```python
from build123d import *

# Parameters (mm, degrees)
F0_W     = 60
F0_H     = 40
F0_R     = 1.75
F0_W_2   = 29
F0_H_2   = 22
F1_DEPTH = 3
F2_R     = 5


with BuildPart() as f1:
    # F0 (on Top) → F1 (new body)
    with BuildSketch(Plane.XY):
        Rectangle(F0_W, F0_H)
        with Locations((-25, 0)):
            Circle(F0_R, mode=Mode.SUBTRACT)
        Rectangle(F0_W_2, F0_H_2, mode=Mode.SUBTRACT)
        with Locations((25, 0)):
            Circle(F0_R, mode=Mode.SUBTRACT)
    extrude(amount=F1_DEPTH)

    # F2
    f2_edges = [f1.edges().sort_by_distance(p)[0] for p in [
        (-30, -20, 1.5),
        (-30, 20, 1.5),
        (30, 20, 1.5),
        (30, -20, 1.5),
    ]]
    fillet(f2_edges, radius=F2_R)


solid = f1.part
```
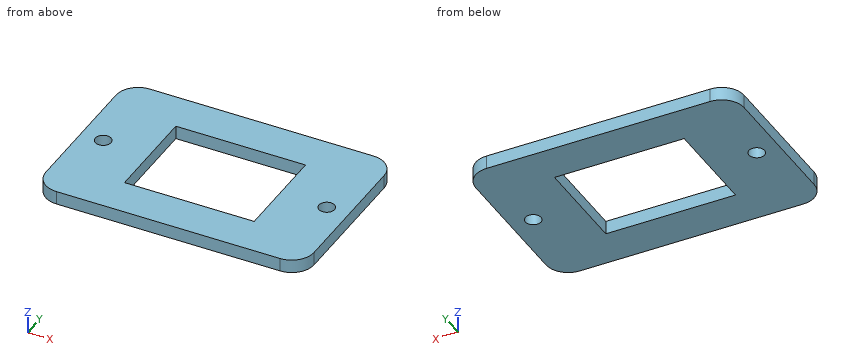
CAD build for the part. Positions are in the model's coordinates, mm. Give positions to 0.01 mm unless a question says otherwise; leave off trailing zeros. Loops run counter-clockwise (first coordinate to the right, second up) from the corner with the lowest first, then second, coordinate; pieces in that order, holes last. Notation, with made-up numbers: M 60.25,25 L 95.25,25 A34 ccw 95.25,59 Z; hole C 27,24 d10. An arc over 180 degrees is marked long. Use one line per item in the form item = value.
Item 1: Slice it at D-D (y = 0). List the corners of the cut face in (x, z).
Determined:
outline = M -30,0 L -26.75,0 L -26.75,3 L -30,3 Z; M -23.25,0 L -14.5,0 L -14.5,3 L -23.25,3 Z; M 14.5,0 L 23.25,0 L 23.25,3 L 14.5,3 Z; M 26.75,0 L 30,0 L 30,3 L 26.75,3 Z
Item 2: Slice it at A-A (z = 1.5). List the corners of the cut face in (x, y).
Determined:
outline = M -30,-15 A5 ccw -25,-20 L 25,-20 A5 ccw 30,-15 L 30,15 A5 ccw 25,20 L -25,20 A5 ccw -30,15 Z; hole C -25,0 d3.5; hole M -14.5,-11 L 14.5,-11 L 14.5,11 L -14.5,11 Z; hole C 25,0 d3.5
Item 3: Drill centre lines: probe 1 along Y at (x, z) = (9.5, 1.5); probe 2 along X at (y, z) = (4, 2.3); probe 3 along Y at (x, z) = (-25, 0.8). Where is each one in solid material? Low to high. Write a range as from..to.
Determined:
probe_1 = -20..-11, 11..20
probe_2 = -30..-14.5, 14.5..30
probe_3 = -20..-1.75, 1.75..20
Item 4: Slice it at B-B (y = -7). List the corners of the cut face in (x, z).
Determined:
outline = M -30,0 L -14.5,0 L -14.5,3 L -30,3 Z; M 14.5,0 L 30,0 L 30,3 L 14.5,3 Z
Item 5: Slice it at C-C (x = 13.5). List the corners of the cut face in (y, z), plus the area to 3 significant figures.
Determined:
outline = M -20,0 L -11,0 L -11,3 L -20,3 Z; M 11,0 L 20,0 L 20,3 L 11,3 Z
area = 54.0 mm2
